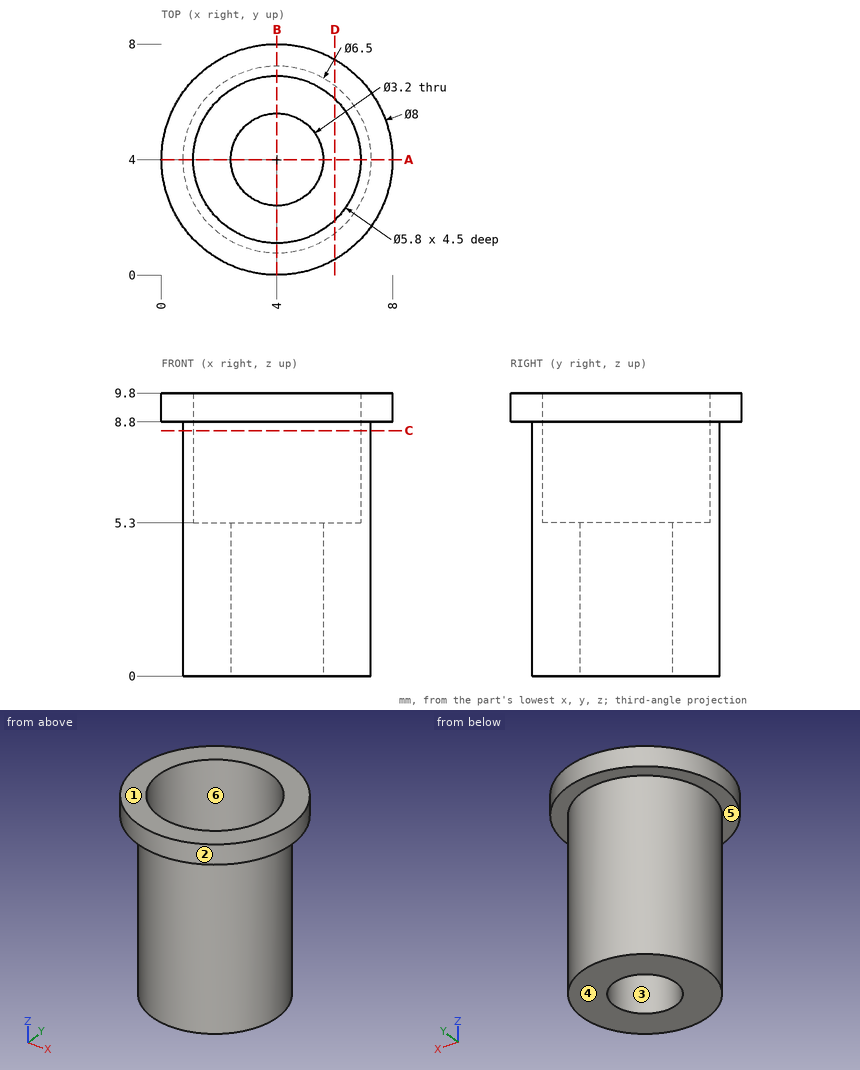
Geometry check sheet. Reference: drawing and pictorial views, mm from the part's lowest x, y, z. A direction names the side the tool comes from. Give positions to 0.01 mm unless a question says otherwise; leave off trailing zeros. Order: outer loops, then holes, each group sorted by start corner. A loop starts at its lowest first (then second) coordinate and runs counter-clockwise, first axis right, second up. Notation, with made-up numbers: M -26,80 L 5,80 A9 cw 5,92 Z; hole C -22.75,15.5 d4. An arc over 180 degrees is marked long. Answer as CSV lines item,"result". Start each with the question number.
Item 1: Cross-section at D-D on x = 6. Enter the section's corners in (y, z).
Item 2: Cross-section at A-A on y = 4. Enter the section's corners in (x, z).
Item 3: Thickness scan on line 1 (Y direction, x = 4, z = 2.5); line 2 (Y direction, x = 4, z = 7.3); line 3 (Z direction, x = 0.5, y = 5.5). Record the ranges inside material, lowest first. Write a range as [from, to].
Item 4: Cross-section at C-C on z = 8.5. Enter the section's corners in (x, y), plus the area to 3 significant figures.
Item 5: Gauge pin test, flat ends, axial feed: P1, Ø4, axis at y = 5, z = 2.5, coming from the +X side; P2, Ø1.5, axis at y = 7, z = 4, coming from the +X side; P3, Ø1.5, axis at x = 3.5, z = 3.5, coming from the -Y side. Record the tip position at first contact, or that the pin passes through.
Item 6: Tool access check on the marked faces 4, 5 and 6. Record the directions out of +Z, -Z, +X, -X, +Y, -Y that give a thin tool (end or side, any length) a straight path to the whole face; none if there is none.
Item 7: Mould release check, pull along Y, two halves, no side actions. Record for the marked faces 1, 2 and 3: +Y half, -Y half, draft (parallel to the pull), parting line (faces both ways), or undercut.
Established:
1,outline,"M 0.54,8.8 L 1.44,8.8 L 1.44,0 L 6.56,0 L 6.56,8.8 L 7.46,8.8 L 7.46,9.8 L 6.1,9.8 L 6.1,5.3 L 1.9,5.3 L 1.9,9.8 L 0.54,9.8 Z"
2,outline,"M 0,8.8 L 0.75,8.8 L 0.75,0 L 2.4,0 L 2.4,5.3 L 1.1,5.3 L 1.1,9.8 L 0,9.8 Z; M 5.6,0 L 7.25,0 L 7.25,8.8 L 8,8.8 L 8,9.8 L 6.9,9.8 L 6.9,5.3 L 5.6,5.3 Z"
3,line 1,"y = [0.75, 2.4], [5.6, 7.25]"
3,line 2,"y = [0.75, 1.1], [6.9, 7.25]"
3,line 3,"z = [8.8, 9.8]"
4,outline,"C 4,4 d6.5; hole C 4,4 d5.8"
4,area,"6.76 mm^2"
5,P1,"stops at x = 7.25"
5,P2,"stops at x = 6.35"
5,P3,"stops at y = 0.75"
6,face 4,"-Z, +X, -X, +Y, -Y"
6,face 5,"-Z"
6,face 6,"+Z"
7,face 1,"draft"
7,face 2,"parting line"
7,face 3,"undercut"
